from build123d import *

# Parameters (mm, degrees)
EXTRUDE_1_DEPTH             = 20
SKETCH_2_R                  = 7
CUT_EXTRUDE_1_DEPTH         = 20
SKETCH_3_R                  = 13
CUT_EXTRUDE_2_DEPTH         = 87.740993769
SKETCH_4_R                  = 16
CUT_EXTRUDE_3_DEPTH         = 19
CUT_EXTRUDE_9_DEPTH         = 87.740993769
EXTRUDE_START               = -20
EXTRUDE_4_DEPTH             = 20
FILLET_2_R                  = 3
SKETCH_7_R                  = 20.5
CUT_EXTRUDE_10_DEPTH        = 9
SKETCH_8_W                  = 29.8
SKETCH_8_H                  = 4
CUT_EXTRUDE_11_DEPTH        = 20
CUT_EXTRUDE_12_DEPTH        = 10
HOLE_WIZARD_M41_D           = 4.3
HOLE_WIZARD_M41_DEPTH       = 8
HOLE_WIZARD_M41_CBORE_D     = 8
HOLE_WIZARD_M41_CBORE_DEPTH = 4.5
M4X0_71_D                   = 3.3


# Read off the part's stored shape, not the designer's step: Бобышка-Вытянуть4
with BuildPart() as part:
    # Эскиз1 → Бобышка-Вытянуть1 (new body)
    with BuildSketch(Plane(origin=(0, 0, 0), x_dir=(1, 0, 0), z_dir=(0, 1, 0))):
        with BuildLine():
            Line((0, 0), (0, 50))
            Line((0, 50), (20, 50))
            Line((20, 50), (47.60878471, 47.400960405))
            ThreePointArc((47.60878471, 47.400960405), (68, 25), (47.60878471, 2.599039595))
            Line((47.60878471, 2.599039595), (20, 0))
            Line((20, 0), (0, 0))
        make_face()
    extrude(amount=EXTRUDE_1_DEPTH)

    # Эскиз2 → Вырез-Вытянуть1 (cut)
    with BuildSketch(Plane.ZY):
        with Locations((-39.9, 10)):
            Circle(SKETCH_2_R)
        with Locations(Location((-10.1, 10, 0), (0, 0, 180))):
            Circle(SKETCH_2_R)
    extrude(amount=-CUT_EXTRUDE_1_DEPTH, mode=Mode.SUBTRACT)

    # Эскиз3 → Вырез-Вытянуть2 (cut, through all)
    with BuildSketch(Plane(origin=(0, 20, 0), x_dir=(1, 0, 0), z_dir=(0, 1, 0))):
        with Locations(Location((45.5, 25, 0), (0, 0, 270))):
            Circle(SKETCH_3_R)
    extrude(amount=-CUT_EXTRUDE_2_DEPTH, mode=Mode.SUBTRACT)

    # Эскиз4 → Вырез-Вытянуть3 (cut)
    with BuildSketch(Plane(origin=(0, 20, 0), x_dir=(1, 0, 0), z_dir=(0, 1, 0))):
        with Locations(Location((45.5, 25, 0), (0, 0, 270))):
            Circle(SKETCH_4_R)
    extrude(amount=-CUT_EXTRUDE_3_DEPTH, mode=Mode.SUBTRACT)

    # Эскиз5 → Вырез-Вытянуть9 (cut, through all)
    with BuildSketch(Plane(origin=(0, 20, 0), x_dir=(1, 0, 0), z_dir=(0, 1, 0))):
        with BuildLine():
            add(Edge.make_bspline(
                [(47.32108314, 47.428044097), (47.41641101, 47.41948544), (47.512308925, 47.410461109), (47.60878471, 47.400960405)],
                knots=[0.992066387, 0.992066387, 0.992066387, 0.992066387, 1, 1, 1, 1], degree=3))
            Line((47.32108314, 47.428044095), (47.60878471, 47.400960405))
        make_face()
        with BuildLine():
            Line((47.32108314, 47.428044097), (23, 49.717585585))
            add(Edge.make_bspline(
                [(23, 49.717585585), (32.393861284, 42.286998451), (35.400716473, 48.498269788), (47.32108314, 47.428044097)],
                knots=[0, 0, 0, 0, 0.992066387, 0.992066387, 0.992066387, 0.992066387], degree=3))
        make_face()
        with BuildLine():
            add(Edge.make_bspline(
                [(23, 0.282414415), (32.393861284, 7.713001549), (35.400716473, 1.501730212), (47.32108314, 2.571955903)],
                knots=[0, 0, 0, 0, 0.992066387, 0.992066387, 0.992066387, 0.992066387], degree=3))
            Line((23, 0.282414415), (47.32108314, 2.571955903))
        make_face()
        with BuildLine():
            Line((47.60878471, 2.599039595), (47.32108314, 2.571955905))
            add(Edge.make_bspline(
                [(47.32108314, 2.571955903), (47.41641101, 2.58051456), (47.512308925, 2.589538891), (47.60878471, 2.599039595)],
                knots=[0.992066387, 0.992066387, 0.992066387, 0.992066387, 1, 1, 1, 1], degree=3))
        make_face()
    extrude(amount=-CUT_EXTRUDE_9_DEPTH, mode=Mode.SUBTRACT)

    # Бобышка-Вытянуть4 outline → Бобышка-Вытянуть4 (add)
    with BuildSketch(Plane(origin=(0, 20, 0), x_dir=(1, 0, 0), z_dir=(0, 1, 0)).offset(EXTRUDE_START)):
        with BuildLine():
            add(Edge.make_bspline(
                [(22.6429674, 50), (22.761978267, 49.905861862), (22.880989133, 49.811723723), (23, 49.717585585)],
                knots=[-0.012568493, -0.012568493, -0.012568493, -0.012568493, 0, 0, 0, 0], degree=3))
            Line((22.6429674, 50), (20, 50))
            Line((20, 50), (23, 49.717585585))
        make_face()
        with BuildLine():
            Line((20, 0), (22.6479861, 0))
            add(Edge.make_bspline(
                [(22.6479861, 0), (22.766323231, 0.09625734), (22.883651508, 0.190382227), (23, 0.282414415)],
                knots=[-0.012287325, -0.012287325, -0.012287325, -0.012287325, 0, 0, 0, 0], degree=3))
            Line((23, 0.282414415), (20, 0))
        make_face()
    extrude(amount=EXTRUDE_4_DEPTH)

    # Скругление2
    fillet_2_edges = [part.edges().sort_by_distance(p)[0] for p in [
        (11.32399305, 0, 0),
        (11.32399305, 20, 0),
        (11.3214837, 0, -50),
        (11.3214837, 20, -50),
    ]]
    fillet(fillet_2_edges, radius=FILLET_2_R)

    # Эскиз7 → Вырез-Вытянуть10 (cut)
    with BuildSketch(Plane(origin=(0, 20, 0), x_dir=(1, 0, 0), z_dir=(0, 1, 0))):
        with Locations(Location((45.5, 25, 0), (0, 0, 270))):
            Circle(SKETCH_7_R)
    extrude(amount=-CUT_EXTRUDE_10_DEPTH, mode=Mode.SUBTRACT)

    # Эскиз8 → Вырез-Вытянуть11 (cut)
    with BuildSketch(Plane.ZY):
        with Locations((-25, 10)):
            Rectangle(SKETCH_8_W, SKETCH_8_H)
    extrude(amount=-CUT_EXTRUDE_11_DEPTH, mode=Mode.SUBTRACT)

    # Эскиз9 → Вырез-Вытянуть12 (cut)
    with BuildSketch(Plane(origin=(0, 20, 0), x_dir=(1, 0, 0), z_dir=(0, 1, 0))):
        with BuildLine():
            Line((20, 39.9), (20, 10.1))
            ThreePointArc((20, 10.1), (18.5, 8.6), (17, 10.1))
            Line((17, 10.1), (17, 39.9))
            ThreePointArc((17, 39.9), (18.5, 41.4), (20, 39.9))
        make_face()
    extrude(amount=-CUT_EXTRUDE_12_DEPTH, mode=Mode.SUBTRACT)

    # Цековка для винта с внутренним шестигранником M41
    with Locations(Plane(origin=(0, 20, 0), x_dir=(1, 0, 0), z_dir=(0, 1, 0))):
        with Locations((8.5, 25)):
            CounterBoreHole(HOLE_WIZARD_M41_D / 2, HOLE_WIZARD_M41_CBORE_D / 2, HOLE_WIZARD_M41_CBORE_DEPTH, depth=HOLE_WIZARD_M41_DEPTH)

    # Отверстие обработанное метчиком M4x0.71 (through all)
    with Locations(Plane(origin=(0, 8, 0), x_dir=(1, 0, 0), z_dir=(0, 1, 0))):
        with Locations((8.5, 25)):
            Hole(M4X0_71_D / 2)


solid = part.part
Model file for the job. Use its own axes, mm. A direction names the side the tool comes from. Round coordinates to 2 decimals unless told otherwise and drop trailing zeros. Order: outer loops, then holes, each group sorted by start corner. A loop starts at its lowest first (then second) coordinate and runs counter-clockwise, first axis right, second up.
(1) Pull direction Z, two halves, no side cores. Call faces 4 (the face through (68, 10, -25)), 5 (the face through (27, 0, -25)), 6 (the face through (13.47, 0.86, -49.1)), 7 (the face through (9.86, 10.279, -46.894)): released by +Z, released by -Z, zero draft, split by the parting line, or undercut.
(2) Band-saw the part on B-B (z = -11). List the corners of the cut face in (x, y).
(3) Drill centre lines: line 1 (X direction, y = 12.9, z = -25); line 2 (X direction, y = 0.55, z = -25); line 3 (X direction, y = 9.5, z = -25.5). Where is each one in solid material? Low to high.
(4) Pin check, flat tips, straight feed: pin 1 (2.5 mm diameter, centred on x = 9, z = -26, fed in from +Y); pin 2 (3 mm diameter, centred on x = 46, z = -11.5, fed in from +Y); pin 3 (8 mm diameter, centred on x = 57, y = 8, fed in from +Z); pin 4 (5 mm diameter, centred on x = 11, z = -22.5, fed in from +Y). Stop position of each tip, or through.
(5) Band-saw the part on D-D (x = 18.5). List the corners of the cut face in (y, z).
(6) Band-saw the part on C-C (z = -35). List the corners of the cut face in (x, y), then the cut area to 3 significant figures.
(7) Band-saw the part on A-A (x = 8.5). List the corners of the cut face in (y, z).
(8) 3-axis set-ups, long thin cutter, end or side, ignore diameter. For faces 1 (the face through (10, 8, -23)), 2 (the face through (56.46, 0.51, -18.01)), 3 (the face through (33, 11, -36)): which of +Z, -Z, +X, -X, +Y, -Y reach the whole face in a straight line?
Verdict:
1. face 4: split by the parting line
1. face 5: zero draft
1. face 6: released by -Z
1. face 7: undercut
2. outline: (0, 0) - (63.11, 0) - (63.11, 20) - (60.47, 20) - (60.47, 11) - (53.25, 11) - (53.25, 1) - (37.75, 1) - (37.75, 11) - (30.53, 11) - (30.53, 20) - (20, 20) - (20, 3.06) - (0, 3.06) - close; (0, 16.94) - (17, 16.94) - (17, 20) - (0, 20) - close
3. line 1: x = 0 to 6.35, 10.65 to 17, 20 to 25, 66 to 68
3. line 2: x = 0 to 6.85, 10.15 to 32.5, 58.5 to 68
3. line 3: x = 20 to 29.51, 61.49 to 67.99
4. pin 1: stops at y = 15.5
4. pin 2: stops at y = 1
4. pin 3: stops at z = -3.79
4. pin 4: stops at y = 20
5. outline: (0, -47) arc R3 ccw to (3, -50) - (17, -50) arc R3 ccw to (20, -47) - (20, -41.4) - (16.84, -41.4) arc R7 cw (long way) to (8, -33.19) - (8, -16.81) arc R7 cw (long way) to (16.84, -8.6) - (20, -8.6) - (20, -3) arc R3 ccw to (17, 0) - (3, 0) arc R3 ccw to (0, -3) - close
6. outline: (0, 0) - (37.19, 0) - (37.19, 1) - (33.01, 1) - (33.01, 11) - (27.6, 11) - (27.6, 20) - (20, 20) - (20, 5) - (0, 5) - close; (0, 15) - (17, 15) - (17, 20) - (0, 20) - close; (53.81, 0) - (65.66, 0) - (65.66, 20) - (63.4, 20) - (63.4, 11) - (57.99, 11) - (57.99, 1) - (53.81, 1) - close
6. area: 510 mm2
7. outline: (0, -47) arc R3 ccw to (3, -50) - (17, -50) arc R3 ccw to (20, -47) - (20, -29) - (15.5, -29) - (15.5, -27.15) - (12, -27.15) - (12, -33.19) arc R7 cw (long way) to (8, -33.19) - (8, -26.65) - (0, -26.65) - close; (0, -23.35) - (8, -23.35) - (8, -16.81) arc R7 cw (long way) to (12, -16.81) - (12, -22.85) - (15.5, -22.85) - (15.5, -21) - (20, -21) - (20, -3) arc R3 ccw to (17, 0) - (3, 0) arc R3 ccw to (0, -3) - close
8. face 1: -X
8. face 2: +Y, -Y
8. face 3: +Y
